```python
from build123d import *

# Parameters (mm, degrees)
F1_R      = 8.5
F2_DEPTH  = 8.375
F4_DEPTH  = 25
F5_R      = 9.25
F6_DEPTH  = 25
F8_R      = 10
F9_DEPTH  = 25
F11_R     = 10
F12_DEPTH = 25
F14_W     = 6.35
F14_H     = 15
F15_DEPTH = 25


with BuildPart() as f2:
    # F1 (on Front) → F2 (new body, symmetric)
    with BuildSketch(Plane.XZ):
        with BuildLine():
            Line((10, 16.5), (-10, 16.5))
            add(Edge.make_bspline(
                [(-9.4202485093, -6.596129018), (-10.7339585576, -4.7199566312), (-13.237953942, 0.2165761702), (-11.6404121135, 10.3778986471), (-10, 16.5)],
                knots=[0, 0, 0, 0, 0.3953497888, 1, 1, 1, 1], degree=3))
            ThreePointArc((-9.4202485093, -6.596129018), (0, -11.5), (9.4202485093, -6.596129018))
            add(Edge.make_bspline(
                [(9.4202485093, -6.596129018), (10.7339585576, -4.7199566312), (13.237953942, 0.2165761702), (11.6404121135, 10.3778986471), (10, 16.5)],
                knots=[0, 0, 0, 0, 0.3953497888, 1, 1, 1, 1], degree=3))
        make_face()
        Circle(F1_R, mode=Mode.SUBTRACT)
    extrude(amount=F2_DEPTH, both=True)

    # F3 (on Right) → F4 (intersect, symmetric)
    with BuildSketch(Plane.YZ):
        with BuildLine():
            Line((0, 23.2340655672), (-7.3927235128, 16.5))
            add(Edge.make_bspline(
                [(-7.3927235128, 16.5), (-7.6966545202, 14.0246805856), (-9.6172618847, 7.6235921039), (-6.1354099401, -2.8855319888), (-3, -11.5)],
                knots=[0, 0, 0, 0, 0.3841811099, 1, 1, 1, 1], degree=3))
            Line((-3, -11.5), (0, -19.7424322584))
            Line((0, -19.7424322584), (3, -11.5))
            add(Edge.make_bspline(
                [(7.3927235128, 16.5), (7.6966545202, 14.0246805856), (9.6172618847, 7.6235921039), (6.1354099401, -2.8855319888), (3, -11.5)],
                knots=[0, 0, 0, 0, 0.3841811099, 1, 1, 1, 1], degree=3))
            Line((7.3927235128, 16.5), (0, 23.2340655672))
        make_face()
    extrude(amount=F4_DEPTH, both=True, mode=Mode.INTERSECT)

    # F5 (on Front) → F6 (cut, symmetric)
    with BuildSketch(Plane.XZ):
        Circle(F5_R)
    extrude(amount=F6_DEPTH, both=True, mode=Mode.SUBTRACT)

    # F8 (on offset) → F9 (cut)
    with BuildSketch(Plane.XZ.offset(2.5)):
        Circle(F8_R)
    extrude(amount=F9_DEPTH, mode=Mode.SUBTRACT)

    # F11 (on offset) → F12 (cut)
    with BuildSketch(Plane.XZ.offset(-2.5)):
        Circle(F11_R)
    extrude(amount=-F12_DEPTH, mode=Mode.SUBTRACT)

    # F14 (on Right) → F15 (cut, symmetric)
    with BuildSketch(Plane.YZ):
        with Locations((0, 19)):
            Rectangle(F14_W, F14_H)
    extrude(amount=F15_DEPTH, both=True, mode=Mode.SUBTRACT)


solid = f2.part
```
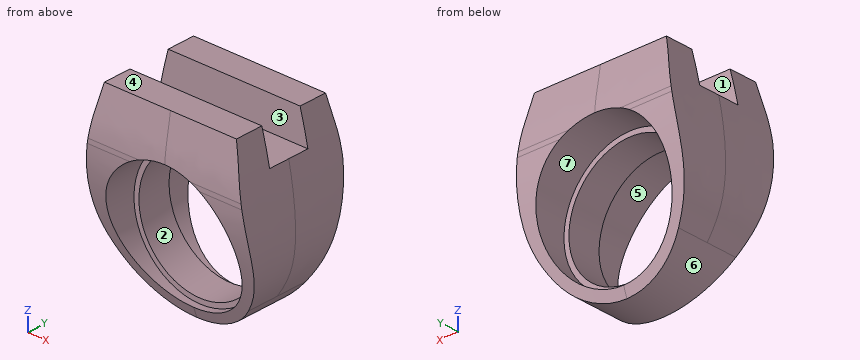
Check sheet for the modelled part. Datum: model origin and axes. Units: mm. Face numbers are marked on the shaded views. A direction names the side the tool comes from. Give positions to 0.01 mm unless a question says otherwise; leave off trailing zeros. Answer in a Markdown table with one row per item.
1) Depth check by flat-ended pin: pin 1 (5 mm diameter, centred on x = -9, y = -5.5, fed in from -Z); pin 2 (3 mm diameter, centred on x = 6.5, y = -5, fed in from -Z); pin 3 (4 mm diameter, centred on y = -6.5, z = -3.5, fed in from +X) (3 decimals). Enter the tip coordinate at first touch or a pass-through.
Solutions:
| item | result |
|---|---|
| pin 1 | stops at z = -9.05 |
| pin 2 | stops at z = -9.84 |
| pin 3 | stops at x = 11.805 |
2) Tool access check on the marked faces 3, 4, 5, 6 and 7. Record the directions out of +Z, -Z, +X, -X, +Y, -Y that give a thin tool (end or side, any length) a straight path to the whole face; none if there is none.
Solutions:
| item | result |
|---|---|
| face 3 | +Z, +X, -X |
| face 4 | +Z, +X, -X, +Y, -Y |
| face 5 | -Y |
| face 6 | -Z, +Y, -Y |
| face 7 | +Y |
3) Thickness scan on line 1 (Z direction, x = 0, y = -1); line 2 (Z direction, x = 0, y = 6.75); line 3 (Z direction, x = 7, y = 0.5). Record the ranges inside material, lowest first.
Solutions:
| item | result |
|---|---|
| line 1 | z = -11.5 to -9.25, 9.25 to 11.5 |
| line 2 | z = 10 to 16.5 |
| line 3 | z = -9.12 to -6.05, 6.05 to 11.5 |
4) Mould release check, pull along Y, two halves, no side actions. Record for the marked faces 1 and 2: released by +Y, released by -Y, zero draft, split by the parting line, or undercut.
Solutions:
| item | result |
|---|---|
| face 1 | undercut |
| face 2 | zero draft |
